Could you check a few things on this model? Use its own coordinates, in mm. A direction names the side the tool comes from. Coordinates: 2 decimals unless noted, no trailing zeros. Loops run counter-clockwise (first coordinate to the right, second up) from the corner with the lowest first, then second, coordinate; pieces in that order, holes last. Notation, with made-up numbers: (-28.75, 48) - (2.25, 48) arc R20 ccw to (2.25, 84) - close; hole circle Ø1 at (64.25, -0.75). An arc over 180 degrees is marked (long way). Use CSV: the item, a comma, the result in double quotes.
from build123d import *

# Parameters (mm, degrees)
SKETCH1_W           = 32
SKETCH1_H           = 17
BOSS_EXTRUDE1_DEPTH = 12
SKETCH2_W           = 15
SKETCH2_H           = 10
CUT_EXTRUDE1_DEPTH  = 58
BOSS_EXTRUDE2_DEPTH = 5
CUT_EXTRUDE2_DEPTH  = 3
SKETCH5_R           = 1.75
CUT_EXTRUDE3_DEPTH  = 4


with BuildPart() as part:
    # Sketch1 → Boss-Extrude1 (new body)
    with BuildSketch(Plane(origin=(0, 0, 0), x_dir=(1, 0, 0), z_dir=(0, 1, 0))):
        Rectangle(SKETCH1_W, SKETCH1_H)
    extrude(amount=BOSS_EXTRUDE1_DEPTH)

    # Sketch2 → Cut-Extrude1 (cut)
    with BuildSketch(Plane.ZY.offset(16)):
        with Locations((0, 5)):
            Rectangle(SKETCH2_W, SKETCH2_H)
    extrude(amount=-CUT_EXTRUDE1_DEPTH, mode=Mode.SUBTRACT)

    # Sketch3 → Boss-Extrude2 (add)
    with BuildSketch(Plane.XZ):
        Polygon((4.330127019, -8.5), (-4.330127019, -8.5), (-8.660254038, -16), (-4.330127019, -23.5), (4.330127019, -23.5), (8.660254038, -16), align=None)
        Polygon((8.660254038, 16), (4.330127019, 8.5), (-4.330127019, 8.5), (-8.660254038, 16), (-4.330127019, 23.5), (4.330127019, 23.5), align=None)
    extrude(amount=-BOSS_EXTRUDE2_DEPTH)

    # Sketch4 → Cut-Extrude2 (cut)
    with BuildSketch(Plane(origin=(0, 5, 0), x_dir=(1, 0, 0), z_dir=(0, 1, 0))):
        Polygon((2.886751346, 11), (5.773502692, 16), (2.886751346, 21), (-2.886751346, 21), (-5.773502692, 16), (-2.886751346, 11), align=None)
        Polygon((2.886751346, -21), (5.773502692, -16), (2.886751346, -11), (-2.886751346, -11), (-5.773502692, -16), (-2.886751346, -21), align=None)
    extrude(amount=-CUT_EXTRUDE2_DEPTH, mode=Mode.SUBTRACT)

    # Sketch5 → Cut-Extrude3 (cut)
    with BuildSketch(Plane(origin=(0, 2, 0), x_dir=(1, 0, 0), z_dir=(0, 1, 0))):
        with Locations(Location((0, 16, 0), (0, 0, 270))):
            Circle(SKETCH5_R)
        with Locations(Location((0, -16, 0), (0, 0, 270))):
            Circle(SKETCH5_R)
    extrude(amount=-CUT_EXTRUDE3_DEPTH, mode=Mode.SUBTRACT)


solid = part.part
(1) Thinking about a two-plate mould opening in Z: for faces 5 (the face through (0, 5, -7.5)), 6 (the face through (0, 2, -23.5)), 7 (the face through (0, 0, 14)), 8 (the face through (4.35, 3.521, 13.535)), which applies, +Z half, -Z half, draft (parallel to the pull), parting line (faces both ways), or undercut?
Computed:
face 5,"undercut"
face 6,"-Z half"
face 7,"draft"
face 8,"undercut"
(2) Suppose I cut it at B-B (x = 0). Write out the boundary of the cut face in (y, z), plus the area to 3 significant figures.
Computed:
outline,"(0, -23.5) - (5, -23.5) - (5, -21) - (2, -21) - (2, -17.75) - (0, -17.75) - close; (0, -14.25) - (2, -14.25) - (2, -11) - (5, -11) - (5, -8.5) - (12, -8.5) - (12, 8.5) - (5, 8.5) - (5, 11) - (2, 11) - (2, 14.25) - (0, 14.25) - (0, 7.5) - (10, 7.5) - (10, -7.5) - (0, -7.5) - close; (0, 17.75) - (2, 17.75) - (2, 21) - (5, 21) - (5, 23.5) - (0, 23.5) - close"
area,"130 mm²"
(3) Please list where these lines run through material, in increasing order: line 1 (Z direction, x = 2.5, y = 4); line 2 (Z direction, x = -11, y = 2); line 3 (X direction, y = 0.75, z = -16).
Computed:
line 1,"z = -23.5 to -21, -11 to -7.5, 7.5 to 11, 21 to 23.5"
line 2,"z = -8.5 to -7.5, 7.5 to 8.5"
line 3,"x = -8.66 to -1.75, 1.75 to 8.66"
(4) Which directions (+Z, -Z, +X, -X, +Y, -Y) give clear straight access to the entire face, cutting with the end or side of a thin tool? Please do faces 1 (the face through (4.35, 3.521, -18.465)), 2 (the face through (6.526, 2.465, 12.302)), 3 (the face through (-6.465, 2.465, -12.198)), 4 (the face through (0, 10, 0)).
Computed:
face 1,"+Y"
face 2,"+X, +Y, -Y"
face 3,"-X, +Y, -Y"
face 4,"+X, -X, -Y"
(5) Suppose I cut it at A-A (y = 1). Write out the boundary of the cut face in (x, z), plus the area to 3 significant figures.
Computed:
outline,"(-16, -8.5) - (-4.33, -8.5) - (-8.66, -16) - (-4.33, -23.5) - (4.33, -23.5) - (8.66, -16) - (4.33, -8.5) - (16, -8.5) - (16, -7.5) - (-16, -7.5) - close; (-16, 7.5) - (16, 7.5) - (16, 8.5) - (4.33, 8.5) - (8.66, 16) - (4.33, 23.5) - (-4.33, 23.5) - (-8.66, 16) - (-4.33, 8.5) - (-16, 8.5) - close; hole circle Ø3.5 at (0, -16); hole circle Ø3.5 at (0, 16)"
area,"434 mm²"
(6) Suppose I cut it at D-D (x = -13.5). Write out the boundary of the cut face in (y, z), plus the area to 3 significant figures.
Computed:
outline,"(0, -8.5) - (12, -8.5) - (12, 8.5) - (0, 8.5) - (0, 7.5) - (10, 7.5) - (10, -7.5) - (0, -7.5) - close"
area,"54.0 mm²"
(7) Will these pins go through, and if not, where does the flat tip stop? pin 1 (4.5 mm diameter, centred on x = 0.5, z = 17, fed in from +Y); pin 2 (3 mm diameter, centred on x = 0, z = -16, fed in from +Y); pin 3 (8 mm diameter, centred on x = 1.5, z = 14.5, fed in from +Y); pin 4 (5 mm diameter, centred on y = 4, z = -16, fed in from +X).
Computed:
pin 1,"stops at y = 2"
pin 2,"passes through"
pin 3,"stops at y = 5"
pin 4,"stops at x = 8.66"
(8) Suppose I cut it at C-C (y = 7). Write out the boundary of the cut face in (x, z).
Computed:
outline,"(-16, -8.5) - (16, -8.5) - (16, -7.5) - (-16, -7.5) - close; (-16, 7.5) - (16, 7.5) - (16, 8.5) - (-16, 8.5) - close"
